from build123d import *

# Parameters (mm, degrees)
STOCK_BEE_ZERKER_START                       = 9.525
STOCK_BEE_ZERKER_2_0_MULTIBODY_1_OUTLINE_R   = 3.175
STOCK_BEE_ZERKER_2_0_MULTIBODY_1_OUTLINE_R_2 = 2.38125
STOCK_BEE_ZERKER_2_0_MULTIBODY_1_DEPTH       = 6.35
FILLET1_R                                    = 0.635
FILLET2_R                                    = 25.4


# Read off the part's stored shape, not the designer's step: Stock-Bee-zerker 2.0 Multibody-1
with BuildPart() as part:
    # Stock-Bee-zerker 2.0 Multibody-1 outline → Stock-Bee-zerker 2.0 Multibody-1 (new body)
    with BuildSketch(Plane.YZ.offset(STOCK_BEE_ZERKER_START)):
        Polygon((0, 63.5), (1.143, 38.33622), (2.667, 38.33622), (2.667, 39.92372), (30.58384403, 39.92372), (6.35, 68.804490685), (6.35, 89.907129746), (9.525, 89.347291582), (0, 109.77372), align=None)
        with Locations((11.1125, 46.27372)):
            Circle(STOCK_BEE_ZERKER_2_0_MULTIBODY_1_OUTLINE_R, mode=Mode.SUBTRACT)
        with Locations((7.818068754, 55.210853084)):
            Circle(STOCK_BEE_ZERKER_2_0_MULTIBODY_1_OUTLINE_R_2, mode=Mode.SUBTRACT)
    extrude(amount=STOCK_BEE_ZERKER_2_0_MULTIBODY_1_DEPTH)

    # Fillet1
    fillet1_edges = [part.edges().sort_by_distance(p)[0] for p in [
        (12.7, 6.35, 89.907129746),
        (12.7, 30.58384403, 39.92372),
        (12.7, 2.667, 39.92372),
        (12.7, 2.667, 38.33622),
        (12.7, 1.143, 38.33622),
    ]]
    fillet(fillet1_edges, radius=FILLET1_R)

    # Fillet2
    # the kernel refuses this fillet: 25.4 mm, written as the material it adds along each edge
    with BuildSketch(Plane(origin=(9.525, 6.35, 68.804490685), x_dir=(0, 0, 1), z_dir=(1, 0, 0))) as fillet2_piece_1:
        with BuildLine():
            CenterArc((FILLET2_R * 0.363970234267, -FILLET2_R), FILLET2_R, 90, 40)
            Line((-FILLET2_R * 0.278817375421, -FILLET2_R * 0.233955556882), (0, 0))
            Line((0, 0), (FILLET2_R * 0.363970234267, 0))
        make_face()
    extrude(amount=6.35)
    # the kernel refuses this fillet: 25.4 mm, written as the material it takes off along each edge
    with BuildSketch(Plane(origin=(8.083580992, 0, 63.5), x_dir=(0, 0.0453756432593108, -0.9989699950442975), z_dir=(1, 0, 0))) as fillet2_2_piece_1:
        with BuildLine():
            CenterArc((FILLET2_R * 0.0226995119346, FILLET2_R), FILLET2_R, 267.399274167, 2.600725833)
            Line((-FILLET2_R * 0.0226761313248, FILLET2_R * 0.0010300049557), (0, 0))
            Line((0, 0), (FILLET2_R * 0.0226995119345, 0))
        make_face()
    extrude(amount=9.232838016, mode=Mode.SUBTRACT)


solid = part.part
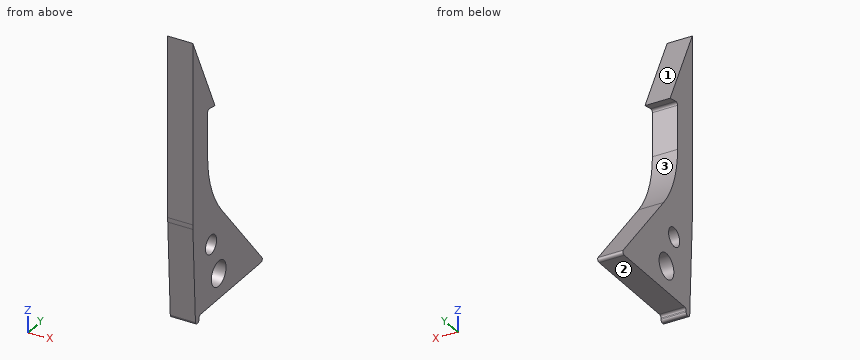
Check sheet for the modelled part. Datum: model origin and axes. Units: mm. Face numbers are marked on the shaded views. A direction names the side the tool comes from. Coordinates: 2 decimals unless noted, no trailing zeros. Write each loop counter-clockwise with the first axis right and the second up, starting at its lowest first coordinate (ties: lowest second). Pieces come first, ordered by that corner, then holes.
Item 1: Cross-section at D-D on z = 56. Record the boundary of the cut face in (x, y) (3 decimals).
Numbers:
outline: (9.525, 0.341) - (15.875, 0.341) - (15.875, 5.571) - (9.525, 5.571) - close; (9.525, 10.065) - (15.875, 10.065) - (15.875, 17.094) - (9.525, 17.094) - close
Item 2: Depth check by flat-ended pin: pin 1 Ø1.9 at (x, y) = (13, 19.5) entering from -Z; pin 2 Ø1.5 at (x, z) = (11, 87) entering from +Y. Enter the tip coordinate at first touch or a pass-through.
Numbers:
pin 1: stops at z = 39.92
pin 2: stops at y = 6.35
Item 3: Scan lines: probe 1 along Y at (x, z) = (14.5, 77.5); probe 2 along Z at (x, y) = (11, 6); probe 3 along Y at (x, z) = (14, 54.5). Record each from-to range of solid material in increasing order.
Numbers:
probe 1: y = 0 to 6.36
probe 2: z = 39.92 to 53.67, 56.75 to 96.91
probe 3: y = 0.41 to 5.55, 10.09 to 18.35
Item 4: Cross-section at A-A on y = 8.75. Record the boundary of the cut face in (x, z) (3 decimals), then the cut area to 3 significant figures.
Numbers:
outline: (9.525, 39.924) - (15.875, 39.924) - (15.875, 44.153) - (9.525, 44.153) - close; (9.525, 48.395) - (15.875, 48.395) - (15.875, 53.02) - (9.525, 53.02) - close; (9.525, 57.402) - (15.875, 57.402) - (15.875, 67.272) - (9.525, 67.272) - close; (9.525, 89.484) - (15.875, 89.484) - (15.875, 91.009) - (9.525, 91.009) - close
area: 129 mm2
Item 5: Cross-section at B-B on z = 48.5. Record the boundary of the cut face in (x, y) (1 decimal).
Numbers:
outline: (9.5, 0.7) - (15.9, 0.7) - (15.9, 8.8) - (9.5, 8.8) - close; (9.5, 13.4) - (15.9, 13.4) - (15.9, 23.4) - (9.5, 23.4) - close
Item 6: Cross-section at C-C on x = 14.5. Count the separate pieces of the cut face and the enclosed holes in it, then the cut area to 3 significant figures.
Numbers:
separate pieces: 1
enclosed holes: 2
area: 710 mm2
Item 7: Access from +Z, -Z, +X, -X, +Y, -Y to the whole of each face (thin tool, end or side, straight path). Record for the marked faces 1, 2 and 3.
Numbers:
face 1: +Z, +X, -X, +Y
face 2: -Z, +X, -X, +Y
face 3: +X, -X, +Y
